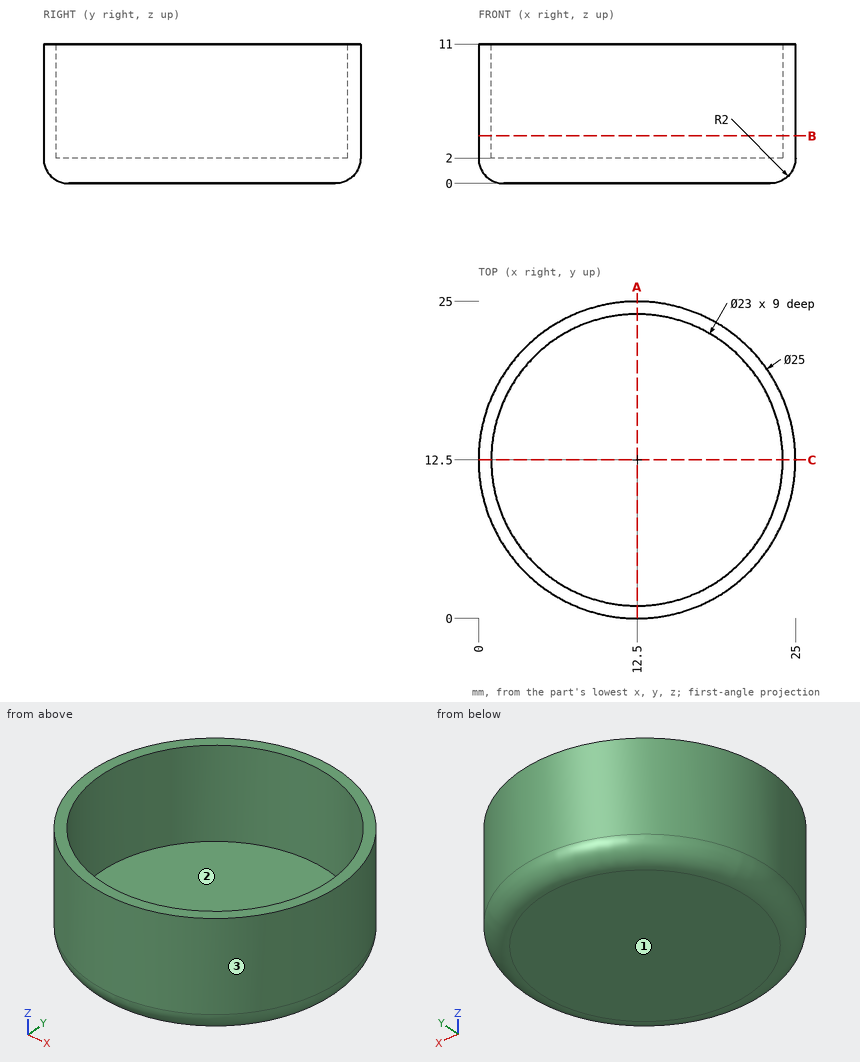
Study the drawing (mm; zero at the part's minimum x, y, z) and answer. Give positions to 0.01 mm unless a question says otherwise; leave off trailing zeros. Write each loop counter-clockwise with the first axis right and the second up, starting at its lowest first coordinate (ties: lowest second). Pieces come first, ordered by that corner, then holes. Notation, with made-up numbers: (58.5, 26) -> (112.5, 26) arc R20 ccw to (112.5, 43) -> close; hole circle Ø1 at (-31, 12.5). An arc over 180 degrees is marked (long way). Answer as a JSON object with one key per item and string values. Group by question number.
1) The mould has two halves that part along Y. Classify the marked faces 1, 2 and 3: +Y half, -Y half, draft (parallel to the pull), parting line (faces both ways), or undercut.
2) Find section A-A (x = 12.5). Write down the section's boundary in (y, z), and give its area (3 significant figures).
3) Each of these flat-tipped pins is pushed along its axis until it touches: P1, Ø3, axis at y = 20.5, z = 2, coming from the -X side; P2, Ø6, axis at x = 7, z = 7.5, coming from the -Y side; P3, Ø7, axis at x = 14, y = 12.5, coming from the +Z side. Where does it stop, or does it pass through?
4) Consider L1, parallel to Y at x = 12.5, z = 8.25; L2, parallel to Z at x = 5, y = 17.75; L3, parallel to Y at x = 20.5, z = 5.5. Determine where each line is inside the solid, lowest interval first. Write a range as from..to.
5) Find section B-B (z = 3.75). Write down the section's boundary in (x, y), and give its area (3 significant figures).
Values follow:
{
 "1": {"face 1": "draft", "face 2": "undercut", "face 3": "parting line"},
 "2": {"outline": "(0, 2) arc R2 ccw to (2, 0) -> (23, 0) arc R2 ccw to (25, 2) -> (25, 11) -> (24, 11) -> (24, 2) -> (1, 2) -> (1, 11) -> (0, 11) -> close", "area": "66.3 mm2"},
 "3": {"P1": "stops at x = 1.82", "P2": "stops at y = 0.25", "P3": "stops at z = 2"},
 "4": {"L1": "y = 0..1, 24..25", "L2": "z = 0..2", "L3": "y = 2.9..4.24, 20.76..22.1"},
 "5": {"outline": "circle Ø25 at (12.5, 12.5); hole circle Ø23 at (12.5, 12.5)", "area": "75.4 mm2"}
}
